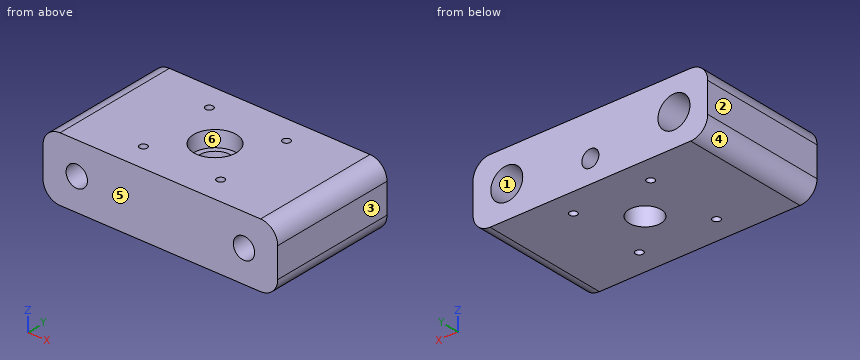
```python
from build123d import *

# Parameters (mm, degrees)
SKETCH1_W           = 69.85
SKETCH1_H           = 38.1
BOSS_EXTRUDE1_DEPTH = 9.525
SKETCH2_R           = 6.35
CUT_EXTRUDE1_DEPTH  = 4.7625
SKETCH3_R           = 4.7625
CUT_EXTRUDE2_DEPTH  = 20.05
SKETCH4_R           = 1.1303
CUT_EXTRUDE3_DEPTH  = 20.05
SKETCH6_R           = 3.175
CUT_EXTRUDE4_DEPTH  = 39.1
SKETCH7_R           = 4.7625
CUT_EXTRUDE5_DEPTH  = 28.575
SKETCH8_R           = 2.54
CUT_EXTRUDE6_DEPTH  = 9.652
FILLET1_R           = 5.08


with BuildPart() as part:
    # Sketch1 → Boss-Extrude1 (new body, symmetric)
    with BuildSketch(Plane.XY):
        with Locations((34.925, 19.05)):
            Rectangle(SKETCH1_W, SKETCH1_H)
    extrude(amount=BOSS_EXTRUDE1_DEPTH, both=True)

    # Sketch2 → Cut-Extrude1 (cut)
    with BuildSketch(Plane.XY.offset(9.525)):
        with Locations((34.925, 19.05)):
            Circle(SKETCH2_R)
    extrude(amount=-CUT_EXTRUDE1_DEPTH, mode=Mode.SUBTRACT)

    # Sketch3 → Cut-Extrude2 (cut, through all)
    with BuildSketch(Plane.XY.offset(9.525)):
        with Locations((34.925, 19.05)):
            Circle(SKETCH3_R)
    extrude(amount=-CUT_EXTRUDE2_DEPTH, mode=Mode.SUBTRACT)

    # Sketch4 → Cut-Extrude3 (cut, through all)
    with BuildSketch(Plane.XY.offset(9.525)):
        with Locations((23.4315, 30.5435)):
            Circle(SKETCH4_R)
        with Locations((46.4185, 30.5435)):
            Circle(SKETCH4_R)
        with Locations((46.4185, 7.5565)):
            Circle(SKETCH4_R)
        with Locations((23.4315, 7.5565)):
            Circle(SKETCH4_R)
    extrude(amount=-CUT_EXTRUDE3_DEPTH, mode=Mode.SUBTRACT)

    # Sketch6 → Cut-Extrude4 (cut, through all)
    with BuildSketch(Plane(origin=(0, 38.1, 0), x_dir=(1, 0, 0), z_dir=(0, 1, 0))):
        with Locations((10.045078415, 0)):
            Circle(SKETCH6_R)
    cut_extrude4 = extrude(amount=-CUT_EXTRUDE4_DEPTH, mode=Mode.SUBTRACT)

    # Sketch7 → Cut-Extrude5 (cut)
    with BuildSketch(Plane(origin=(0, 38.1, 0), x_dir=(1, 0, 0), z_dir=(0, 1, 0))):
        with Locations((10.045078415, 0)):
            Circle(SKETCH7_R)
    cut_extrude5 = extrude(amount=-CUT_EXTRUDE5_DEPTH, mode=Mode.SUBTRACT)

    # Mirror1: Cut-Extrude4, Cut-Extrude5 across plane
    add(cut_extrude4.mirror(Plane.ZY.offset(-34.925)), mode=Mode.SUBTRACT)
    add(cut_extrude5.mirror(Plane.ZY.offset(-34.925)), mode=Mode.SUBTRACT)

    # Sketch8 → Cut-Extrude6 (cut)
    with BuildSketch(Plane(origin=(0, 38.1, 0), x_dir=(1, 0, 0), z_dir=(0, 1, 0))):
        with Locations((34.925, 2.788579275)):
            Circle(SKETCH8_R)
    extrude(amount=-CUT_EXTRUDE6_DEPTH, mode=Mode.SUBTRACT)

    # Fillet1
    fillet1_edges = [part.edges().sort_by_distance(p)[0] for p in [
        (69.85, 19.05, 9.525),
        (0, 19.05, 9.525),
        (69.85, 19.05, -9.525),
        (0, 19.05, -9.525),
    ]]
    fillet(fillet1_edges, radius=FILLET1_R)


solid = part.part
```
Could you check a few things on this model? Use its own coordinates, in mm. Face numbers are marked on the shaded views. A direction names the side the tool comes from. Round coordinates to 2 decimals unless told otherwise and drop trailing zeros. Write each loop counter-clockwise with the first axis right and the second up, starting at its lowest first coordinate (ties: lowest second). Pieces come first, ordered by that corner, then holes. Notation, with made-up numbers: M -22.75,45 L -10.75,45 A7 cw -10.75,56 Z; hole C -11,6 d8. An arc over 180 degrees is marked long. Answer in a Markdown table with one row per item. Add a question column.
Q1. Imagine slicing it at B-B (y = 4). Please give me the cut outline in (x, z) (3 decimals), then the cut area to 3 significant figures.
Q2. If I drill on line 1 (X direction, y = 31.75, z = 0); line 2 (X direction, y = 34.5, z = 4); line 3 (X direction, y = 31, z = 0.25), over which ranges is the centre line in solid material (lowest first)? Write a range as from..to.
Q3. Will these pins go through, and if not, where does the flat tip stop? pin 1 Ø1.5 at (x, z) = (34, -3.5) entering from +Y; pin 2 Ø4 at (y, z) = (14.5, -7) entering from -X; pin 3 Ø1 at (y, z) = (15.5, 7.5) entering from +X.
Q4. On a 3-axis mill with a long thin cutter (end or side, diameter ignored), from which of +Z, -Z, +X, -X, +Y, -Y can I reach the whole of each face in a straight line? I mean the marked faces 1 and 2. Say none if no direction works.
Q5. If we mould it in two halves opening along X, with no side actions, what happens to the marked faces 3, 4, 5 and 6? For each: +X half, -X half, draft (parallel to the pull), parting line (faces both ways), or undercut.
Q6. Imagine slicing it at C-C (x = 11). Please give me the cut outline in (y, z) (3 decimals).
Q7. Imagine slicing it at A-A (y = 19.05). Give the number of separate pieces and of enclosed holes in the cut face, then the cut area to 3 significant figures.
Values:
| question | item | result |
|---|---|---|
| 1 | outline | M 0,-4.445 A5.08 ccw 5.08,-9.525 L 64.77,-9.525 A5.08 ccw 69.85,-4.445 L 69.85,4.445 A5.08 ccw 64.77,9.525 L 5.08,9.525 A5.08 ccw 0,4.445 Z; hole C 10.045,0 d6.35; hole C 59.805,0 d6.35 |
| 1 | area | 1,250 mm^2 |
| 2 | line 1 | 0..5.28, 14.81..55.04, 64.57..69.85 |
| 2 | line 2 | 0..7.46, 12.63..57.22, 62.39..69.85 |
| 2 | line 3 | 0..5.29, 14.8..22.4, 24.47..45.38, 47.45..55.05, 64.56..69.85 |
| 3 | pin 1 | y = 28.45 |
| 3 | pin 2 | x = 0.03 |
| 3 | pin 3 | x = 69.16 |
| 4 | face 1 | +Y |
| 4 | face 2 | +Z, -Z, -X, +Y, -Y |
| 5 | face 3 | +X half |
| 5 | face 4 | -X half |
| 5 | face 5 | draft |
| 5 | face 6 | undercut |
| 6 | outline | M 0,-9.525 L 38.1,-9.525 L 38.1,-4.666 L 9.525,-4.666 L 9.525,-3.028 L 0,-3.028 Z; M 0,3.028 L 9.525,3.028 L 9.525,4.666 L 38.1,4.666 L 38.1,9.525 L 0,9.525 Z |
| 7 | separate pieces | 2 |
| 7 | enclosed holes | 2 |
| 7 | area | 969 mm^2 |
